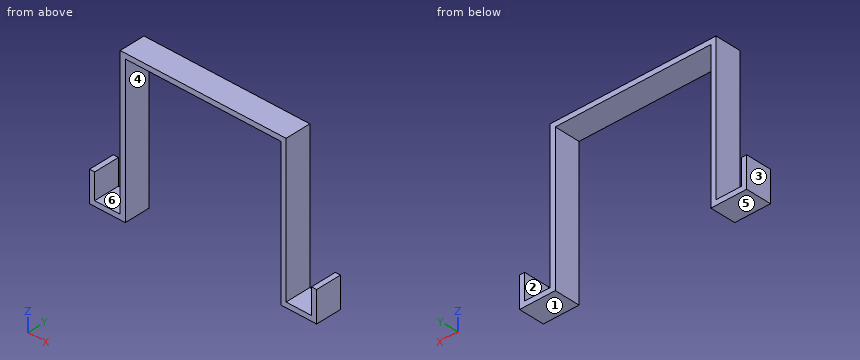
from build123d import *

# Parameters (mm, degrees)
BOSS_EXTRUDE1_DEPTH = 12.7


with BuildPart() as part:
    # Sketch1 → Boss-Extrude1 (new, symmetric)
    with BuildSketch(Plane(origin=(0, 0, 0), x_dir=(1, 0, 0), z_dir=(0, 1, 0))):
        Polygon((-107.95, -25.4), (-107.95, 0), (-82.55, 0), (-82.55, -144.78), (82.55, -144.78), (82.55, 0), (107.95, 0), (107.95, -25.4), (113.03, -25.4), (113.03, 5.08), (77.47, 5.08), (77.47, -139.7), (-77.47, -139.7), (-77.47, 5.08), (-113.03, 5.08), (-113.03, -25.4), align=None)
    extrude(amount=BOSS_EXTRUDE1_DEPTH, both=True)


solid = part.part
Verification items for the finished model (mm, model axes). Face numbers are marked on the shaded views. A direction names the side the tool comes from. Coordinates: 2 decimals unless noted, no trailing zeros. Write each loop counter-clockwise with the first axis right and the second up, starting at its lowest first coordinate (ties: lowest second). Pieces come first, ordered by that corner, then holes. Notation, with made-up numbers: (15, -31) -> (44, -31) arc R17 cw to (44, -14) -> close; hole circle Ø11 at (43.5, 41). An arc over 180 degrees is marked (long way). One line per item, written item: value. Start each with the question number.
Q1. Go/stop test with flat-tipped pins: P1, Ø1.5, axis at x = -65, y = 2, coming from the -Z side; P2, Ø4, axis at y = -8.5, z = 52.5, coming from the +X side; P3, Ø5.5, axis at x = 110.5, y = 5, coming from the +Z side. Record where each tip stops, or that it passes through.
Q2. Cross-section at C-C on x = -73. Enter the section's corners in (y, z), and give its area (3 significant figures).
Q3. Access from +Z, -Z, +X, -X, +Y, -Y to the whole of each face (thin tool, end or side, straight path). Record for the marked faces 4, 5 and 6.
Q4. Mould release check, pull along X, two halves, no side actions. Record for the marked faces 1, 2 and 3: pulls with the +X half, pulls with the -X half, needs draft (parallel to the pull), parting line crosses it, or undercut.
Q5. Cross-section at B-B on y = 8.25. Enter the section's corners in (x, z).
Q6. Cross-section at A-A on z = 107. Enter the section's corners in (x, y), and give its area (3 significant figures).
Q7. Thickness scan on L1, parallel to X at y = 10.75, z = 15.5; L2, parallel to X at y = 9, z = 100; L3, parallel to Z at x = -67.5, y = -8.5. Record the ranges inside material, lowest first. Write a range as from..to.
Checked values:
1. P1: stops at z = 139.7
1. P2: stops at x = 82.55
1. P3: stops at z = 25.4
2. outline: (-12.7, 139.7) -> (12.7, 139.7) -> (12.7, 144.78) -> (-12.7, 144.78) -> close
2. area: 129 mm²
3. face 4: -Z, +Y, -Y
3. face 5: -Z, +X, -X, +Y, -Y
3. face 6: +Z, +Y, -Y
4. face 1: needs draft
4. face 2: undercut
4. face 3: pulls with the -X half
5. outline: (-113.03, -5.08) -> (-77.47, -5.08) -> (-77.47, 139.7) -> (77.47, 139.7) -> (77.47, -5.08) -> (113.03, -5.08) -> (113.03, 25.4) -> (107.95, 25.4) -> (107.95, 0) -> (82.55, 0) -> (82.55, 144.78) -> (-82.55, 144.78) -> (-82.55, 0) -> (-107.95, 0) -> (-107.95, 25.4) -> (-113.03, 25.4) -> close
6. outline: (-82.55, -12.7) -> (-77.47, -12.7) -> (-77.47, 12.7) -> (-82.55, 12.7) -> close; (77.47, -12.7) -> (82.55, -12.7) -> (82.55, 12.7) -> (77.47, 12.7) -> close
6. area: 258 mm²
7. L1: x = -113.03..-107.95, -82.55..-77.47, 77.47..82.55, 107.95..113.03
7. L2: x = -82.55..-77.47, 77.47..82.55
7. L3: z = 139.7..144.78
